Part print with two shaded views. Sizes in mm from the minimum x, y, z corner. Round coordinates to 2 decimals unless told otherwise and drop trailing zeros. Loops run counter-clockwise (first coordinate to the right, second up) from the corner with the lowest first, then second, coordinate; pieces in that order, holes last. Notation, with made-up numbers: (48.25, 63.5) - (86.25, 63.5) arc R12 cw to (86.25, 84.5) - close; hole circle Ø5 at (0.5, -38). An arc over 180 degrees is marked (long way). Put each result on its own line as item: value. Start each with the question number.
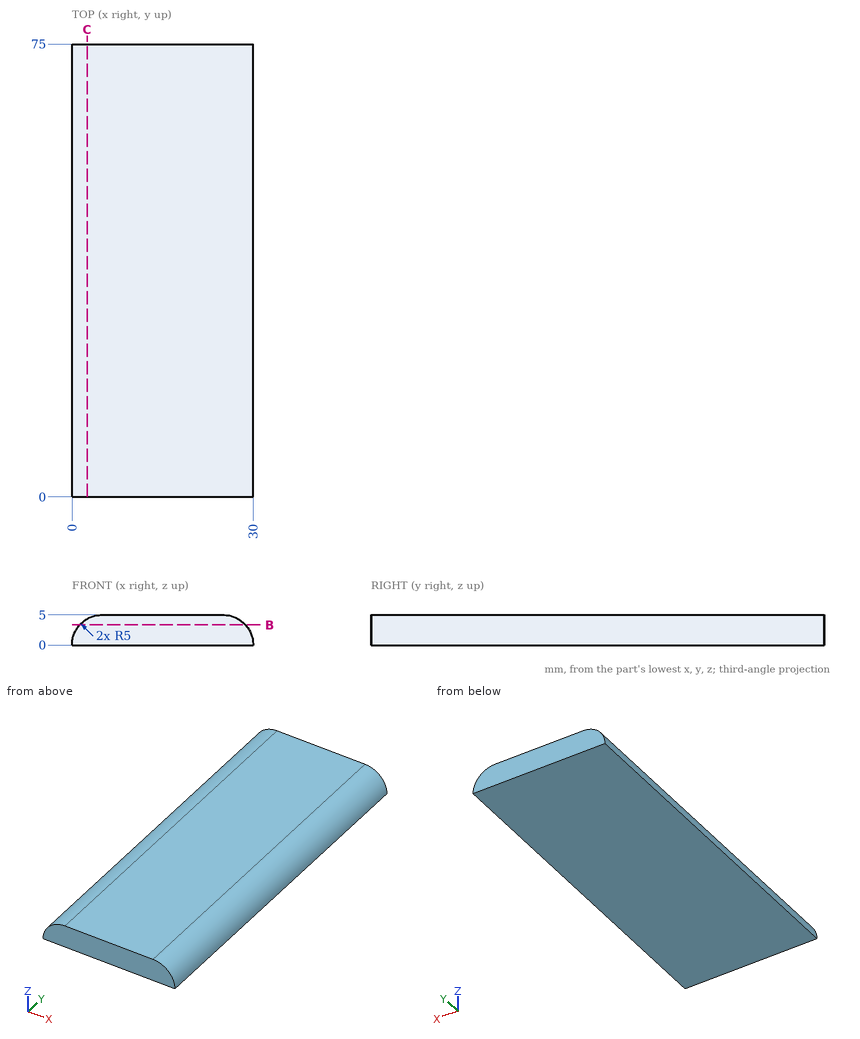
1) Drill centre lines: line 1 (X direction, y = 31, z = 4.1); line 2 (X direction, y = 29, z = 2.9); line 3 (Z direction, x = 2, y = 46.5). Where is each one in solid material? Low to high. Write a range as [from, to].
2) Slice it at B-B, the plane z = 3.35. Write the cut outline in (x, y), and give its area (3 significant figures).
3) Slice it at C-C, the plane x = 2.5. Write the cut outline in (y, z).
Taken from the geometry:
1. line 1: x = [2.14, 27.86]
1. line 2: x = [0.93, 29.07]
1. line 3: z = [0, 4]
2. outline: (1.29, 0) - (28.71, 0) - (28.71, 75) - (1.29, 75) - close
2. area: 2,060 mm2
3. outline: (0, 0) - (75, 0) - (75, 4.33) - (0, 4.33) - close
